The figure shows three views and two pictorial views of one solid part (mm, origin at its lowest corner). Answer the questions. Give positions to 0.01 mm unless a question says otherwise; leave off trailing zeros. Loops run counter-clockwise (first coordinate to the right, second up) from the corner with the lowest first, then second, coordinate; pieces in that order, holes last. Notation, with made-up numbers: (11.25, 8.5) -> (31.25, 8.5) arc R26 ccw to (31.25, 42.5) -> close; hole circle Ø10 at (30.5, 66.5). An arc over 180 degrees is marked (long way). Answer as CSV lines item,"result". Start each with the question number.
1. Find section A-A, the plane z = 5. Give the vertices of the cut face in (x, y).
2. Find section C-C, the plane y = 1.65. Give the vertices of the cut face in (x, z), and give its area (3 significant figures).
3. Find section B-B, the plane x = 5. Give the vertices of the cut face in (y, z).
4. Flat-ended cylindrical pins translate along their axes: pin 1 Ø1.5 at (y, z) = (1.5, 4.5) entering from +X; pin 2 Ø3.5 at (x, z) = (5, 5) entering from +Y. Find the tip coordinate at first contact, or state that the pin passes through.
5. Determine the mould class of the marked faces 1, 2 and 3 for opening direction Z: +Z half, -Z half, draft (parallel to the pull), parting line (faces both ways), or undercut.
6. Find the intervals of material crossed by line 1 along X through (y, z) = (2, 5); line 2 along Z through (x, y) = (4, 2.1), in increasing order.
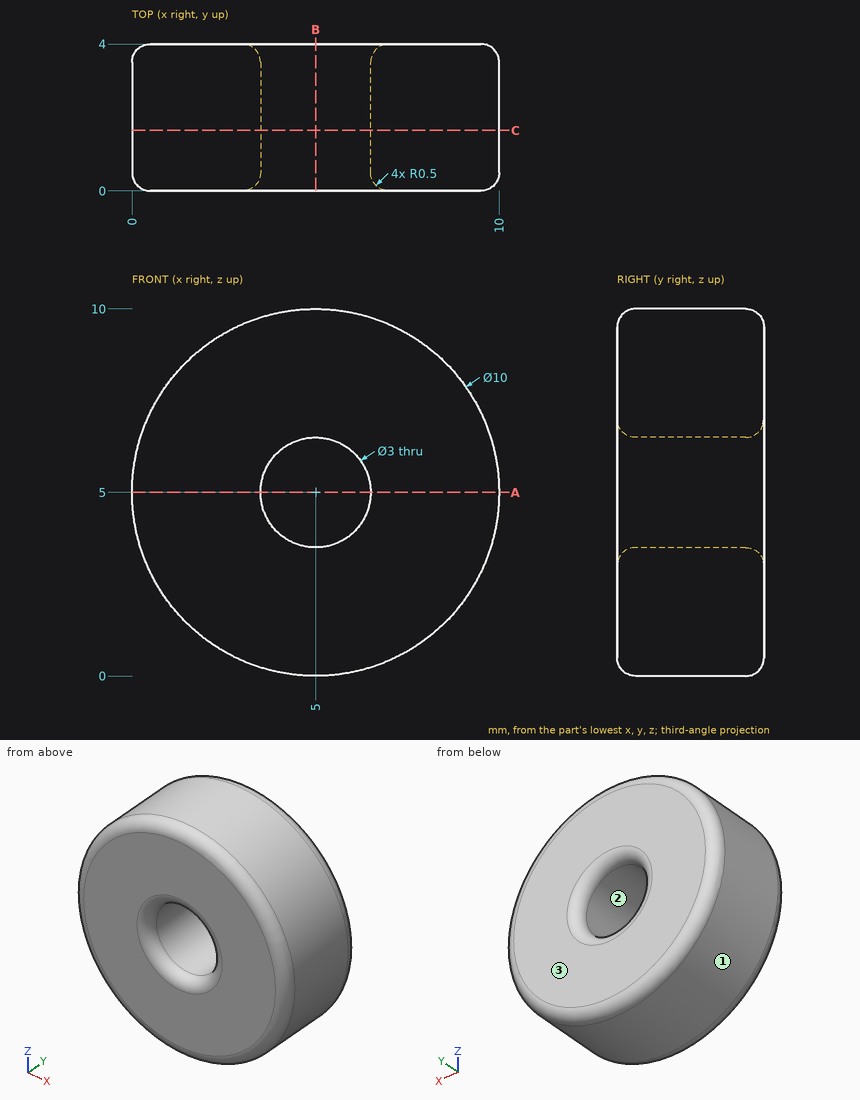
Resolved:
1,outline,"(0, 0.5) arc R0.5 ccw to (0.5, 0) -> (3, 0) arc R0.5 ccw to (3.5, 0.5) -> (3.5, 3.5) arc R0.5 ccw to (3, 4) -> (0.5, 4) arc R0.5 ccw to (0, 3.5) -> close; (6.5, 0.5) arc R0.5 ccw to (7, 0) -> (9.5, 0) arc R0.5 ccw to (10, 0.5) -> (10, 3.5) arc R0.5 ccw to (9.5, 4) -> (7, 4) arc R0.5 ccw to (6.5, 3.5) -> close"
2,outline,"circle Ø10 at (5, 5); hole circle Ø3 at (5, 5)"
2,area,"71.5 mm^2"
3,outline,"(0, 0.5) arc R0.5 ccw to (0.5, 0) -> (3.5, 0) arc R0.5 ccw to (4, 0.5) -> (4, 3) arc R0.5 ccw to (3.5, 3.5) -> (0.5, 3.5) arc R0.5 ccw to (0, 3) -> close; (0, 7) arc R0.5 ccw to (0.5, 6.5) -> (3.5, 6.5) arc R0.5 ccw to (4, 7) -> (4, 9.5) arc R0.5 ccw to (3.5, 10) -> (0.5, 10) arc R0.5 ccw to (0, 9.5) -> close"
4,pin 1,"stops at x = 10"
4,pin 2,"stops at y = 3.93"
5,face 1,"parting line"
5,face 2,"undercut"
5,face 3,"draft"
6,line 1,"x = 0 to 3.5, 6.5 to 10"
6,line 2,"z = 0.1 to 3.88, 6.12 to 9.9"
